Verification items for this drawing (mm, ordinates from the low corner). Give positions to 0.01 mm unless a question says otherwise; leave off trailing zeros. Write each loop counter-clockwise with the first axis right and the second up, starting at its lowest first coordinate (ties: lowest second). Pieces come first, ordered by that corner, then holes. Notation, with made-up numbers: (6, 69.5) -> (54, 69.5) arc R14 ccw to (54, 76.5) -> close; hole circle Ø3 at (17, 44). An arc over 180 degrees is marked (long way). Write item = value, one per line.
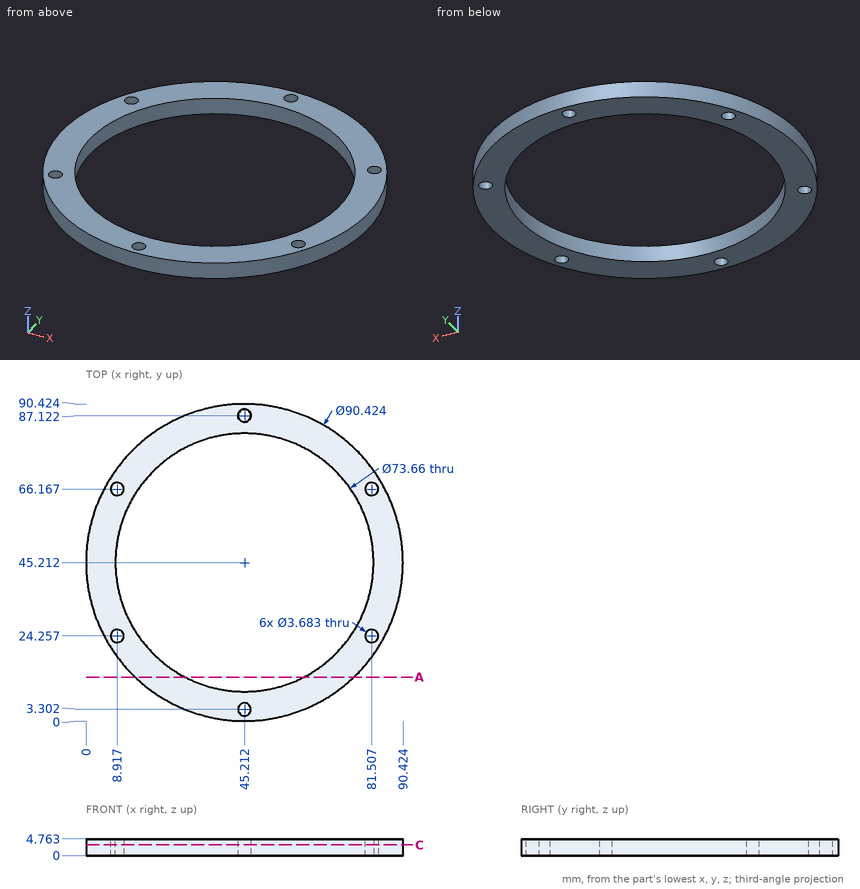
Item 1: Material ranges on line 1 (X direction, y = 45.5, z = 3.8); line 2 (Y direction, x = 11.5, z = 1.1) (1 decimal); line 3 (Y direction, x = 17, z = 4.35) (1 decimal), recorded low to high.
Response values:
line_1 = 0 to 8.38, 82.04 to 90.42
line_2 = 15.1 to 30.4, 60 to 75.3
line_3 = 9.9 to 21.5, 68.9 to 80.5
Item 2: Go/stop test with flat-tipped pins: P1, Ø2, axis at x = 45.212, y = 3.302, coming from the +Z side; P2, Ø1.5, axis at y = 23, z = 3.5, coming from the +X side (1 decimal); P3, Ø1.5, axis at x = 74, z = 2, coming from the -Y side (1 decimal). Record where each tip stops, or that it passes through.
Response values:
P1 = through
P2 = 85
P3 = 9.7
Item 3: Sectioned sample at C-C on z = 3.1. Record the cut outline in (x, y) (1 decimal), then the cut area to 3 significant figures.
Response values:
outline = circle Ø90.4 at (45.2, 45.2); hole circle Ø3.7 at (8.9, 24.3); hole circle Ø3.7 at (8.9, 66.2); hole circle Ø73.7 at (45.2, 45.2); hole circle Ø3.7 at (45.2, 3.3); hole circle Ø3.7 at (45.2, 87.1); hole circle Ø3.7 at (81.5, 24.3); hole circle Ø3.7 at (81.5, 66.2)
area = 2,100 mm^2
Item 4: Sectioned sample at A-A on y = 12.5. Record the cut outline in (x, z) (1 decimal).
Response values:
outline = (14, 0) -> (28.3, 0) -> (28.3, 4.8) -> (14, 4.8) -> close; (62.1, 0) -> (76.4, 0) -> (76.4, 4.8) -> (62.1, 4.8) -> close
